from build123d import *

# Parameters (mm, degrees)
SKETCH1_W                                       = 20
SKETCH1_H                                       = 30
BOSS_EXTRUDE1_DEPTH                             = 3
SKETCH3_R                                       = 3
BOSS_EXTRUDE2_DEPTH                             = 3
FILLET1_R                                       = 2.5
CSK_FOR_M3_FLAT_HEAD_MACHINE_SCREW1_D           = 3.6
CSK_FOR_M3_FLAT_HEAD_MACHINE_SCREW1_DEPTH       = 5
CSK_FOR_M3_FLAT_HEAD_MACHINE_SCREW1_CSINK_D     = 6.3
CSK_FOR_M3_FLAT_HEAD_MACHINE_SCREW1_CSINK_ANGLE = 90
CSK_FOR_M3_FLAT_HEAD_MACHINE_SCREW1_TIP         = 1.081549114
FILLET2_R                                       = 2.5


with BuildPart() as part:
    # Sketch1 → Boss-Extrude1 (new body)
    with BuildSketch(Plane(origin=(0, 0, 0), x_dir=(1, 0, 0), z_dir=(0, 1, 0))):
        Rectangle(SKETCH1_W, SKETCH1_H)
    extrude(amount=BOSS_EXTRUDE1_DEPTH)

    # Sketch3 → Boss-Extrude2 (add)
    with BuildSketch(Plane(origin=(10, 0, 0), x_dir=(0, 0, -1), z_dir=(1, 0, 0))):
        with BuildLine():
            ThreePointArc((-4.472135955, 24.05572809), (0, 26.819660113), (4.472135955, 24.05572809))
            Line((4.472135955, 24.05572809), (15, 3))
            Line((15, 3), (-15, 3))
            Line((-15, 3), (-4.472135955, 24.05572809))
        make_face()
        with Locations((0, 21.819660113)):
            Circle(SKETCH3_R, mode=Mode.SUBTRACT)
    extrude(amount=-BOSS_EXTRUDE2_DEPTH)

    # Fillet1
    fillet1_edges = [part.edges().sort_by_distance(p)[0] for p in [
        (10, 0, 0),
        (-10, 1.5, -15),
        (-10, 1.5, 15),
    ]]
    fillet(fillet1_edges, radius=FILLET1_R)

    # CSK for M3 Flat Head Machine Screw1
    with Locations(Plane(origin=(0, 3, 0), x_dir=(1, 0, 0), z_dir=(0, 1, 0))):
        with Locations((-3, 10), (-3, -10)):
            CounterSinkHole(CSK_FOR_M3_FLAT_HEAD_MACHINE_SCREW1_D / 2, CSK_FOR_M3_FLAT_HEAD_MACHINE_SCREW1_CSINK_D / 2, depth=CSK_FOR_M3_FLAT_HEAD_MACHINE_SCREW1_DEPTH, counter_sink_angle=CSK_FOR_M3_FLAT_HEAD_MACHINE_SCREW1_CSINK_ANGLE)
            with Locations((0, 0, -(CSK_FOR_M3_FLAT_HEAD_MACHINE_SCREW1_DEPTH + CSK_FOR_M3_FLAT_HEAD_MACHINE_SCREW1_TIP / 2))):  # 118° drill point
                Cone(0, CSK_FOR_M3_FLAT_HEAD_MACHINE_SCREW1_D / 2, CSK_FOR_M3_FLAT_HEAD_MACHINE_SCREW1_TIP, mode=Mode.SUBTRACT)

    # Fillet2
    fillet2_edges = [part.edges().sort_by_distance(p)[0] for p in [
        (7, 3, 0),
    ]]
    fillet(fillet2_edges, radius=FILLET2_R)


solid = part.part
Could you check a few things on this model? Use its own coordinates, in mm. A direction names the side the tool comes from. Give positions to 0.01 mm unless a question says otherwise; leave off trailing zeros. Order: outer loops, then holes, each group sorted by start corner. A loop starts at its lowest first (then second) coordinate and runs counter-clockwise, first axis right, second up.
Item 1: For faces 5 (the face through (10, 12, 0)), 6 (the face through (7, 14, 0)), which set-ups out of +Z, -Z, +X, -X, +Y, -Y let a thin tool reach every point of the face, with its end or its side?
Item 2: If we section it at B-B, the plane x = -3: Write out the boundary of the cut face in (y, z), plus the area to 3 significant figures.
Item 3: I'm going to push flat-ended pins straight in: pin 1 (8 mm diameter, centred on y = 20, z = 0.5, fed in from -X); pin 2 (12 mm diameter, centred on x = -3, z = -5.5, fed in from +Y); pin 3 (10 mm diameter, centred on y = 23.5, z = -11, fed in from +X); pin 4 (6 mm diameter, centred on x = -3, z = 10, fed in from +Y). Where does each tip first touch, or does it pass through?
Item 4: I need wall thicknesses on line 1 (Z direction, x = -3, y = 1); line 2 (X direction, y = 10, z = 9); line 3 (Y direction, x = -7.75, z = 14). Which ranges of each line are inside material? Lowest first, please.
Item 5: If we section it at A-A, the plane z = 0: Write out the boundary of the cut face in (x, y).
Item 6: If we section it at D-D, the plane x = 6: Write out the boundary of the cut face in (y, z).
Item 7: If we section it at C-C, the plane y = 20: Write out the boundary of the cut face in (x, z).
Item 8: If we mould it in two halves opening along X, with no side actions, what happens to faces 1 (the face through (-3.831, 0.813, 11.597)), 2 (the face through (-3, 3, 0)), 3 (the face through (9.287, 0.752, -0.21)), 4 (the face through (-3.831, 0.813, -8.403))? For each: pulls with the +X half, pulls with the -X half, needs draft (parallel to the pull), parting line crosses it, or undercut.
Values:
1. face 5: +Z, -Z, +X, +Y, -Y
1. face 6: +Z, -Z, -X, +Y
2. outline: (0, -15) - (3, -15) - (3, -13.15) - (1.65, -11.8) - (0, -11.8) - close; (0, -8.2) - (1.65, -8.2) - (3, -6.85) - (3, 6.85) - (1.65, 8.2) - (0, 8.2) - close; (0, 11.8) - (1.65, 11.8) - (3, 13.15) - (3, 15) - (0, 15) - close
2. area: 64.8 mm2
3. pin 1: stops at x = 7
3. pin 2: stops at y = 3
3. pin 3: passes through
3. pin 4: stops at y = 2.85
4. line 1: z = -15 to -11.8, -8.2 to 8.2, 11.8 to 15
4. line 2: x = 7 to 10
4. line 3: y = 0 to 3
5. outline: (-10, 0) - (7.5, 0) arc R2.5 ccw to (10, 2.5) - (10, 18.82) - (7, 18.82) - (7, 5.5) arc R2.5 cw to (4.5, 3) - (-10, 3) - close; (7, 24.82) - (10, 24.82) - (10, 26.82) - (7, 26.82) - close
6. outline: (0, -15) - (3, -15) - (3.5, -14.75) - (3.5, 14.75) - (3, 15) - (0, 15) - close
7. outline: (7, -6.5) - (10, -6.5) - (10, -2.39) - (7, -2.39) - close; (7, 2.39) - (10, 2.39) - (10, 6.5) - (7, 6.5) - close
8. face 1: undercut
8. face 2: needs draft
8. face 3: pulls with the +X half
8. face 4: undercut
